Could you check a few things on this model? Use its own coordinates, in mm. Face numbers are marked on the shaded views. A direction names the side the tool comes from. Coordinates: 2 decimals unless noted, no trailing zeros. Order: outer loops, then holes, each group sorted by start corner. A loop starts at its lowest first (then second) coordinate and runs counter-clockwise, first axis right, second up. Notation, with made-up numbers: M -25.75,2.25 L -6.75,2.25 A24 cw -6.75,27.25 Z; hole C -20,59.25 d10. An arc over 180 degrees is marked long. Write item = value, one per line. Start each with the question number.
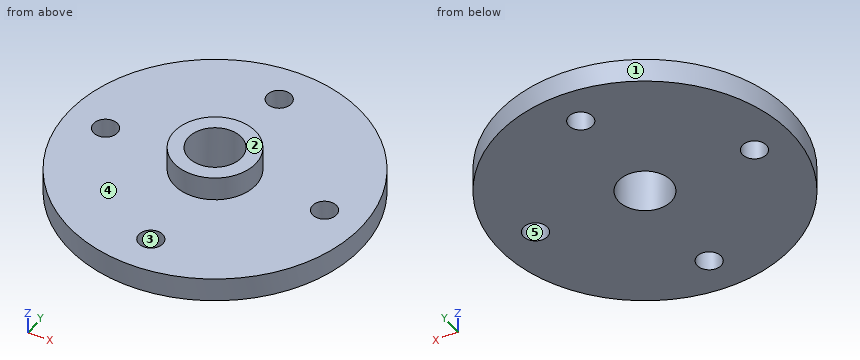
from build123d import *

# Parameters (mm, degrees)
F0_R     = 25.5
F0_R_2   = 8.5
F1_DEPTH = 5
F0_R_3   = 5.5
F2_DEPTH = 10
F3_D     = 5
F0_R_4   = 30.5
F4_DEPTH = 5


# Not quite as in the source:
# - a feature names something its author has since deleted; it is built from what else it names


with BuildPart() as f1:
    # F0 (on Top) → F1 (new body)
    with BuildSketch(Plane.XY):
        Circle(F0_R)
        Circle(F0_R_2, mode=Mode.SUBTRACT)
    extrude(amount=F1_DEPTH)

    # F0 (on Top) → F2 (join)
    with BuildSketch(Plane.XY):
        Circle(F0_R_2)
        Circle(F0_R_3, mode=Mode.SUBTRACT)
    extrude(amount=F2_DEPTH)

    # F3 (through all)
    with Locations(Plane(origin=(0, 0, 0), x_dir=(1, 0, 0), z_dir=(0, 0, -1))):
        with Locations((-22.5, 0), (0, -22.5), (22.5, 0), (0, 22.5)):
            Hole(F3_D / 2)

    # F0 (on Top) → F4 (join, through all)
    with BuildSketch(Plane.XY):
        Circle(F0_R_4)
        Circle(F0_R, mode=Mode.SUBTRACT)
    extrude(amount=F4_DEPTH)


solid = f1.part
(1) Imagine slicing it at D-D on z = 2.5. List the corners of the cut face in (x, y) for me.
(2) Thinking about a two-plate mould opening in Y: for the marked faces 1, 2 and 3, which applies, released by +Y, released by -Y, zero draft, split by the parting line, or undercut?
(3) Please list where these lines run through material, in increasing order: probe 1 along Y at (x, z) = (0, 2.9); probe 2 along Y at (x, z) = (0, 7); probe 3 along Z at (x, y) = (-11.5, 22.5). Write a range as from..to.
(4) Will these pins go through, and if not, where does the flat tip stop? P1, Ø5, axis at x = 13, y = -8, coming from the +Z side; P2, Ø5, axis at x = -5, z = 1.5, coming from the +Y side.
(5) Imagine slicing it at A-A on x = 0. List the corners of the cut face in (y, z) for me.
(6) For the marked faces 4 and 5, which set-ups out of +Z, -Z, +X, -X, +Y, -Y let a thin tool reach every point of the face, with its end or its side?
(7) Imagine slicing it at C-C on y = 22.5. List the corners of the cut face in (x, z) for me, plus the area to 3 significant figures.
Response:
q1.outline = C 0,0 d61; hole C -22.5,0 d5; hole C 0,0 d11; hole C 0,-22.5 d5; hole C 0,22.5 d5; hole C 22.5,0 d5
q2.face_1 = split by the parting line
q2.face_2 = zero draft
q2.face_3 = undercut
q3.probe_1 = -30.5..-25, -20..-5.5, 5.5..20, 25..30.5
q3.probe_2 = -8.5..-5.5, 5.5..8.5
q3.probe_3 = 0..5
q4.P1 = 5
q4.P2 = 30.4
q5.outline = M -30.5,0 L -25,0 L -25,5 L -30.5,5 Z; M -20,0 L -5.5,0 L -5.5,10 L -8.5,10 L -8.5,5 L -20,5 Z; M 5.5,0 L 20,0 L 20,5 L 8.5,5 L 8.5,10 L 5.5,10 Z; M 25,0 L 30.5,0 L 30.5,5 L 25,5 Z
q6.face_4 = +Z
q6.face_5 = +Z, -Z
q7.outline = M -20.59,0 L -2.5,0 L -2.5,5 L -20.59,5 Z; M 2.5,0 L 20.59,0 L 20.59,5 L 2.5,5 Z
q7.area = 181 mm2
